```python
from build123d import *

# Parameters (mm, degrees)
SKETCH1_R           = 1.6
SKETCH1_W           = 20
SKETCH1_H           = 4.5
BOSS_EXTRUDE1_DEPTH = 0.75


with BuildPart() as part:
    # Sketch1 → Boss-Extrude1 (new, symmetric)
    with BuildSketch(Plane.XY):
        with BuildLine():
            Line((-20, 14.2), (-20, -30))
            ThreePointArc((-20, -30), (-15.460155108, -40.960155108), (-4.5, -45.5))
            Line((-4.5, -45.5), (-2.123950753, -45.5))
            Line((-2.123950753, -45.5), (-2.123950753, -43.0422605))
            ThreePointArc((-2.123950753, -43.0422605), (0, -37.625), (2.123950753, -43.0422605))
            Line((2.123950753, -43.0422605), (2.123950753, -45.5))
            Line((2.123950753, -45.5), (4.5, -45.5))
            ThreePointArc((4.5, -45.5), (15.460155108, -40.960155108), (20, -30))
            Line((20, -30), (20, 14.2))
            ThreePointArc((20, 14.2), (18.389087297, 18.089087297), (14.5, 19.7))
            Line((14.5, 19.7), (-14.5, 19.7))
            ThreePointArc((-14.5, 19.7), (-18.389087297, 18.089087297), (-20, 14.2))
        make_face()
        with Locations((-15.25, 15.25)):
            Circle(SKETCH1_R, mode=Mode.SUBTRACT)
        with Locations((15.25, 15.25)):
            Circle(SKETCH1_R, mode=Mode.SUBTRACT)
        with Locations((15.25, -15.25)):
            Circle(SKETCH1_R, mode=Mode.SUBTRACT)
        with Locations((-15.25, -15.25)):
            Circle(SKETCH1_R, mode=Mode.SUBTRACT)
        with Locations((12.75, -30.95)):
            Circle(SKETCH1_R, mode=Mode.SUBTRACT)
        with Locations((-12.75, -30.95)):
            Circle(SKETCH1_R, mode=Mode.SUBTRACT)
        with Locations((0, -22.25)):
            Rectangle(SKETCH1_W, SKETCH1_H, mode=Mode.SUBTRACT)
        with BuildLine():
            Line((-14, 7.5), (-14, -7.5))
            ThreePointArc((-14, -7.5), (-12.622245939, -9.400739328), (-10.387190008, -8.682727327))
            Line((-10.387190008, -8.682727327), (-4.887190008, -1.182727327))
            ThreePointArc((-4.887190008, -1.182727327), (-4.5, 0), (-4.887190008, 1.182727327))
            Line((-4.887190008, 1.182727327), (-10.387190008, 8.682727327))
            ThreePointArc((-10.387190008, 8.682727327), (-12.622245939, 9.400739328), (-14, 7.5))
        make_face(mode=Mode.SUBTRACT)
        with BuildLine():
            Line((4.887190008, 1.182727327), (10.387190008, 8.682727327))
            ThreePointArc((10.387190008, 8.682727327), (12.622245939, 9.400739328), (14, 7.5))
            Line((14, 7.5), (14, -7.5))
            ThreePointArc((14, -7.5), (12.622245939, -9.400739328), (10.387190008, -8.682727327))
            Line((10.387190008, -8.682727327), (4.887190008, -1.182727327))
            ThreePointArc((4.887190008, -1.182727327), (4.5, 0), (4.887190008, 1.182727327))
        make_face(mode=Mode.SUBTRACT)
        with BuildLine():
            Line((-7.897610015, 11.069375575), (-1.397610015, 4.719375575))
            ThreePointArc((-1.397610015, 4.719375575), (0, 4.15), (1.397610015, 4.719375575))
            Line((1.397610015, 4.719375575), (7.897610015, 11.069375575))
            ThreePointArc((7.897610015, 11.069375575), (8.352194489, 13.254569795), (6.5, 14.5))
            Line((6.5, 14.5), (-6.5, 14.5))
            ThreePointArc((-6.5, 14.5), (-8.352194489, 13.254569795), (-7.897610015, 11.069375575))
        make_face(mode=Mode.SUBTRACT)
        with BuildLine():
            Line((6.5, -14.5), (-6.5, -14.5))
            ThreePointArc((-6.5, -14.5), (-8.352194489, -13.254569795), (-7.897610015, -11.069375575))
            Line((-7.897610015, -11.069375575), (-1.397610015, -4.719375575))
            ThreePointArc((-1.397610015, -4.719375575), (0, -4.15), (1.397610015, -4.719375575))
            Line((1.397610015, -4.719375575), (7.897610015, -11.069375575))
            ThreePointArc((7.897610015, -11.069375575), (8.352194489, -13.254569795), (6.5, -14.5))
        make_face(mode=Mode.SUBTRACT)
    extrude(amount=BOSS_EXTRUDE1_DEPTH, both=True)


solid = part.part
```
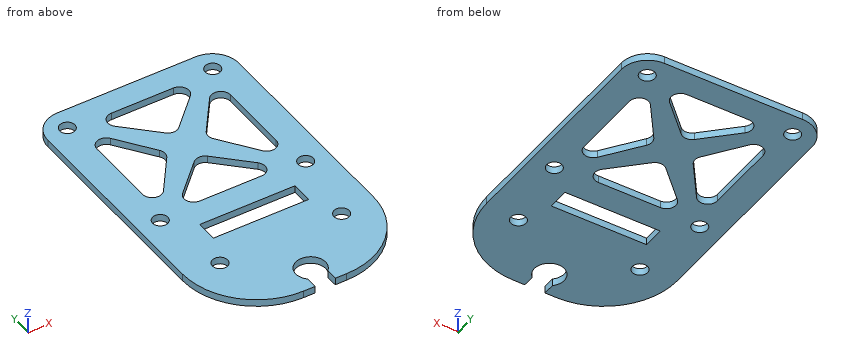
Work out the finished part from the listing and answer in its coordinate system (mm). Round coordinates to 2 decimals unless told otherwise and drop trailing zeros. Order: outer loops, then holes, each group sorted by start corner. A loop starts at its lowest first (then second) coordinate and runs counter-clockwise, first axis right, second up.
Q1. Given pin 1 Ø4 at (x, y) = (-15.25, -15.25) entering from -Z; pin 2 Ø0.8 at (y, z) = (-44, 0.5) entering from +X, each flat-ended and moving along its own axis, determine where each tip first touches the part or whether it passes through.
Solution:
pin 1: stops at z = -0.75
pin 2: stops at x = 11.94
Q2. A cutting plane is placed at D-D, the plane x = 12.75. Determine the outline of the cut face in (y, z), then the cut area to 3 significant figures.
Solution:
outline: (-43.12, -0.75) - (-32.55, -0.75) - (-32.55, 0.75) - (-43.12, 0.75) - close; (-29.35, -0.75) - (-9.35, -0.75) - (-9.35, 0.75) - (-29.35, 0.75) - close; (9.35, -0.75) - (19.7, -0.75) - (19.7, 0.75) - (9.35, 0.75) - close
area: 61.4 mm2
Q3. A cutting plane is placed at A-A, the plane x = 0. Determine the outline of the cut face in (y, z) (3 decimals).
Solution:
outline: (-37.625, -0.75) - (-24.5, -0.75) - (-24.5, 0.75) - (-37.625, 0.75) - close; (-20, -0.75) - (-14.5, -0.75) - (-14.5, 0.75) - (-20, 0.75) - close; (-4.15, -0.75) - (4.15, -0.75) - (4.15, 0.75) - (-4.15, 0.75) - close; (14.5, -0.75) - (19.7, -0.75) - (19.7, 0.75) - (14.5, 0.75) - close
Q4. A cutting plane is placed at B-B, the plane y = -6. Determine the outline of the cut face in (x, z).
Solution:
outline: (-20, -0.75) - (-14, -0.75) - (-14, 0.75) - (-20, 0.75) - close; (-8.42, -0.75) - (-2.71, -0.75) - (-2.71, 0.75) - (-8.42, 0.75) - close; (2.71, -0.75) - (8.42, -0.75) - (8.42, 0.75) - (2.71, 0.75) - close; (14, -0.75) - (20, -0.75) - (20, 0.75) - (14, 0.75) - close
Q5. A cutting plane is placed at C-C, the plane z = -0.5. Count the separate pieces of the cut face and the enclosed holes in it, then the cut area to 3 significant figures.
Solution:
separate pieces: 1
enclosed holes: 11
area: 1,840 mm2
Q6. Find the intervals of material crossed by line 1 along X through (y, z) = (-21, 0.4); line 2 along Y through (x, z) = (-15.5, -0.25); line 3 along Y through (x, z) = (-12.75, -0.2), in increasing order.
Solution:
line 1: x = -20 to -10, 10 to 20
line 2: y = -40.92 to -16.83, -13.67 to 13.67, 16.83 to 19.61
line 3: y = -43.12 to -32.55, -29.35 to -9.35, 9.35 to 19.7
